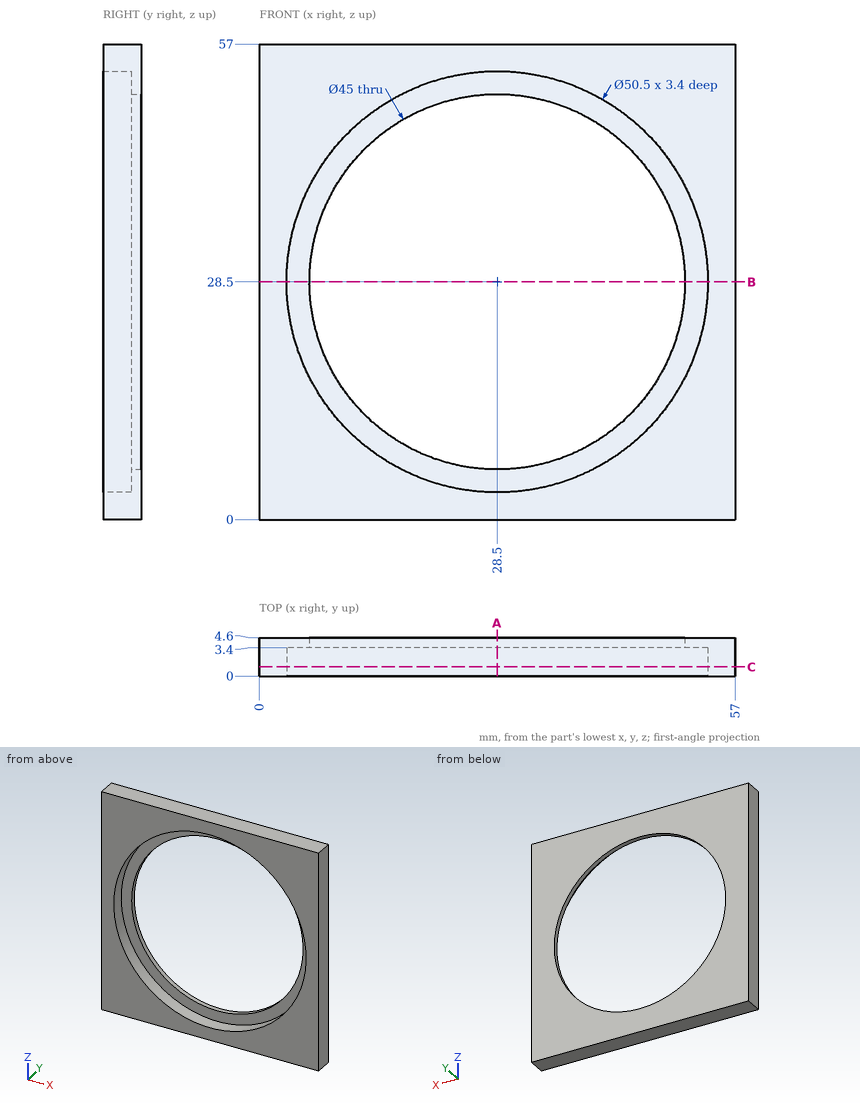
Part print with two shaded views. Sizes in mm from the minimum x, y, z corner. Coordinates: 2 decimals unless noted, no trailing zeros. Order: outer loops, then holes, each group sorted by start corner. A loop starts at its lowest first (then second) coordinate and runs counter-clockwise, first axis right, second up.
(1) Drill centre lines: L1, parallel to X at y = 0.7, z = 28.5; L2, parallel to Z at x = 21, y = 1.45; L3, parallel to Z at x = 32, y = 2.4. Where is each one in solid material? Low to high.
Solution:
L1: x = 0 to 3.25, 53.75 to 57
L2: z = 0 to 4.39, 52.61 to 57
L3: z = 0 to 3.49, 53.51 to 57
(2) Saw through at B-B, the plane z = 28.5. Write the cut outline in (x, y), and give its area (3 significant figures).
Solution:
outline: (0, 0) - (3.25, 0) - (3.25, 3.4) - (6, 3.4) - (6, 4.6) - (0, 4.6) - close; (51, 3.4) - (53.75, 3.4) - (53.75, 0) - (57, 0) - (57, 4.6) - (51, 4.6) - close
area: 36.5 mm2
(3) Saw through at C-C, the plane y = 1.1. Write the cut outline in (x, z), and give its area (3 significant figures).
Solution:
outline: (0, 0) - (57, 0) - (57, 57) - (0, 57) - close; hole circle Ø50.5 at (28.5, 28.5)
area: 1,250 mm2
(4) Saw through at A-A, the plane x = 28.5. Write the cut outline in (y, z).
Solution:
outline: (0, 0) - (4.6, 0) - (4.6, 6) - (3.4, 6) - (3.4, 3.25) - (0, 3.25) - close; (0, 53.75) - (3.4, 53.75) - (3.4, 51) - (4.6, 51) - (4.6, 57) - (0, 57) - close
